For this review, take the finished solid that the model builds, in its own axes (mm). A direction names the side the tool comes from. Give positions to 0.01 mm unless a question says otherwise; leave off trailing zeros. Write each loop counter-clockwise with the first axis right and the second up, starting at its lowest first coordinate (ties: lowest second). Pieces come first, ordered by that corner, then holes. Notation, with made-up numbers: (11, -10.75) -> (50, -10.75) arc R11 ccw to (50, 4.25) -> close; hole circle Ø3 at (34.25, -30.75). An arc over 180 degrees is marked (long way). Write item = value, one per line.
```python
from build123d import *

# Parameters (mm, degrees)
F1_W           = 50
F1_H           = 40
F2_DEPTH       = 10
F3_T1_DEPTH    = 49.9995000031
F6_D           = 5
F6_DEPTH       = 20
F6_CSINK_D     = 10
F6_CSINK_ANGLE = 90
F6_TIP         = 1.5021515476
F7_R           = 2
F8_R           = 12.5
F8_R_2         = 6.5
F9_DEPTH       = 35
F10_DEPTH      = 25


# Not quite as in the source:
# - a fillet or chamfer that OpenCascade refuses, or shapes differently, is made with other operations: its cross-section is extruded or revolved along the edge and cut away or added


with BuildPart() as f2:
    # F1 (on Top) → F2 (new body)
    with BuildSketch(Plane.XY):
        Rectangle(F1_W, F1_H)
    extrude(amount=F2_DEPTH)

    # F3: fillet of radius 8 on 4 edges, made by hand

    # F3_s2 → F3_t1 (cut)
    with BuildSketch(Plane.XY.offset(-19.9997500016)):
        with BuildLine():
            ThreePointArc((-17.0001, 20.0001), (-22.6569542495, 17.6569542495), (-25.0001, 12.0001))
            Line((-25.0001, 12.0001), (-25.1601, 12.0001))
            ThreePointArc((-25.1601, 12.0001), (-25.16, 16.00005), (-25.16, 20))
            Line((-25.16, 20), (-25, 20.16))
            ThreePointArc((-25, 20.16), (-21.00005, 20.16), (-17.0001, 20.1601))
            Line((-17.0001, 20.1601), (-17.0001, 20.0001))
        make_face()
        with BuildLine():
            ThreePointArc((25.0001, 12.0001), (22.6569542495, 17.6569542495), (17.0001, 20.0001))
            Line((17.0001, 20.0001), (17.0001, 20.1601))
            ThreePointArc((17.0001, 20.1601), (21.00005, 20.16), (25, 20.16))
            Line((25, 20.16), (25.16, 20))
            ThreePointArc((25.16, 20), (25.16, 16.00005), (25.1601, 12.0001))
            Line((25.1601, 12.0001), (25.0001, 12.0001))
        make_face()
        with BuildLine():
            ThreePointArc((17.0001, -20.0001), (22.6569542495, -17.6569542495), (25.0001, -12.0001))
            Line((25.0001, -12.0001), (25.1601, -12.0001))
            ThreePointArc((25.1601, -12.0001), (25.16, -16.00005), (25.16, -20))
            Line((25.16, -20), (25, -20.16))
            ThreePointArc((25, -20.16), (21.00005, -20.16), (17.0001, -20.1601))
            Line((17.0001, -20.1601), (17.0001, -20.0001))
        make_face()
        with BuildLine():
            ThreePointArc((-17.0001, -20.0001), (-22.6569542495, -17.6569542495), (-25.0001, -12.0001))
            Line((-25.0001, -12.0001), (-25.1601, -12.0001))
            ThreePointArc((-25.1601, -12.0001), (-25.16, -16.00005), (-25.16, -20))
            Line((-25.16, -20), (-25, -20.16))
            ThreePointArc((-25, -20.16), (-21.00005, -20.16), (-17.0001, -20.1601))
            Line((-17.0001, -20.1601), (-17.0001, -20.0001))
        make_face()
    extrude(amount=F3_T1_DEPTH, mode=Mode.SUBTRACT)

    # F6
    with Locations(Plane(origin=(0, 0, 0), x_dir=(1, 0, 0), z_dir=(0, 0, -1))):
        with Locations((17.5, 12.5), (-17.5, 12.5), (-17.5, -12.5), (17.5, -12.5)):
            CounterSinkHole(F6_D / 2, F6_CSINK_D / 2, depth=F6_DEPTH, counter_sink_angle=F6_CSINK_ANGLE)
            with Locations((0, 0, -(F6_DEPTH + F6_TIP / 2))):  # 118° drill point
                Cone(0, F6_D / 2, F6_TIP, mode=Mode.SUBTRACT)

    # F7
    f7_edges = [f2.edges().sort_by_distance(p)[0] for p in [
        (0, -20, 0),
        (-22.656954, -17.656954, 0),
        (-25, 0, 0),
        (22.656954, -17.656954, 0),
        (-22.656954, 17.656954, 0),
        (25, 0, 0),
        (0, 20, 0),
        (22.656954, 17.656954, 0),
    ]]
    fillet(f7_edges, radius=F7_R)

    # F8 (on face) → F9 (join)
    with BuildSketch(Plane.XY.offset(10)):
        Circle(F8_R)
        Circle(F8_R_2, mode=Mode.SUBTRACT)
    extrude(amount=F9_DEPTH)

    # F10 (cut): a face of the model
    f10_faces = [f2.faces().sort_by_distance(p)[0] for p in [
        (0, 0, 10),
    ]]
    extrude(f10_faces, amount=-F10_DEPTH, mode=Mode.SUBTRACT)


solid = f2.part
```
(1) Tool access review of faces 4 (the face through (22.718, 17.595, 5.944)), 5 (the face through (11.923, 3.755, 27.255)): name each direction out of +Z, -Z, +X, -X, +Y, -Y from which nothing blocks a thin tool from reaching the whole face with its end or side.
Answers below:
face_4 = +Z, -Z, +X, +Y
face_5 = +Z
(2) The part is to be moulded in two halves that separate along X. For faces 1 (the face through (24.43, 0.17, 0.6)), 2 (the face through (19.43, -14.27, 2.38)), 3 (the face through (0, 20, 6)), say which applies: released by +X, released by -X, zero draft, split by the parting line, or undercut.
Answers below:
face_1 = released by +X
face_2 = undercut
face_3 = zero draft
(3) Take a section at D-D (z = 11). Write out the cut boundary in (x, y).
Answers below:
outline = circle Ø25 at (0, 0); hole circle Ø13 at (0, 0)
(4) For pin 1 (1.5 mm diameter, centred on x = -4, z = 27, fed in from +Y); pin 2 (2 mm diameter, centred on y = -15, z = 35.5, fed in from -X); pin 3 (3 mm diameter, centred on x = -9.5, y = 0, fed in from -Z); pin 4 (6 mm diameter, centred on x = -17.5, y = -12.5, fed in from +Z), all flat-tipped, find the tip position at first contact; note any pin that passes through.
Answers below:
pin_1 = 12.07
pin_2 = through
pin_3 = 0
pin_4 = 10
(5) Take a section at B-B (x = 0). Write out the cut boundary in (y, z), plus the area to 3 significant figures.
Answers below:
outline = (-20, 2) arc R2 ccw to (-18, 0) -> (-6.5, 0) -> (-6.5, 45) -> (-12.5, 45) -> (-12.5, 10) -> (-20, 10) -> close; (6.5, 0) -> (18, 0) arc R2 ccw to (20, 2) -> (20, 10) -> (12.5, 10) -> (12.5, 45) -> (6.5, 45) -> close
area = 688 mm^2
(6) Take a section at A-A (y = 0). Write out the cut boundary in (x, z).
Answers below:
outline = (-25, 2) arc R2 ccw to (-23, 0) -> (-6.5, 0) -> (-6.5, 45) -> (-12.5, 45) -> (-12.5, 10) -> (-25, 10) -> close; (6.5, 0) -> (23, 0) arc R2 ccw to (25, 2) -> (25, 10) -> (12.5, 10) -> (12.5, 45) -> (6.5, 45) -> close
(7) To check wall thickness, follow probe 1 along X at (y, z) = (-12.5, 6.5); probe 2 along Y at (x, z) = (17.5, 4.5); probe 3 along Y at (x, z) = (-17, 7). State the ranges of each line that lie inside material, in increasing order.
Answers below:
probe_1 = -24.98 to -20, -15 to 15, 20 to 24.98
probe_2 = -19.98 to -15, -10 to 10, 15 to 19.98
probe_3 = -20 to -14.95, -10.05 to 10.05, 14.95 to 20
(8) Take a section at C-C (z = 4.5). Write out the cut boundary in (x, y), plus the area to 3 significant figures.
Answers below:
outline = (-25, -12.04) arc R8 ccw to (-17.04, -20) -> (17.04, -20) arc R8 ccw to (25, -12.04) -> (25, 12.04) arc R8 ccw to (17.04, 20) -> (-17.04, 20) arc R8 ccw to (-25, 12.04) -> close; hole circle Ø5 at (-17.5, -12.5); hole circle Ø5 at (-17.5, 12.5); hole circle Ø13 at (0, 0); hole circle Ø5 at (17.5, -12.5); hole circle Ø5 at (17.5, 12.5)
area = 1,730 mm^2
